from build123d import *


with BuildPart() as part:
    # 草图1 → 旋转1 (revolve)
    with BuildSketch(Plane.XY, mode=Mode.PRIVATE) as revolve_1_sk:
        Polygon((0, 0), (0, 42), (11.5, 42), (12.5, 40.267949192), (12.5, 0.267949192), (12, 0.267949192), (12, -0.732050808), (7.5, -0.732050808), (7.5, -22.732050808), (6.5, -23.732050808), (0, -23.732050808), align=None)
    revolve(revolve_1_sk.sketch.rotate(Axis((0, 0, 0), (0, 1, 0)), 90), axis=Axis((0, 0, 0), (0, 1, 0)))


solid = part.part
The listing builds one solid part. Answer for the finished solid, in the listing's coordinates (mm). A direction names the side the tool comes from. Round coordinates to 2 decimals unless told otherwise and drop trailing zeros. Write each loop counter-clockwise with the first axis right and the second up, starting at its lowest first coordinate (ties: lowest second). Pieces come first, ordered by that corner, then holes. Notation, with made-up numbers: (31.25, 24.5) - (67.25, 24.5) arc R28 ccw to (67.25, 50.5) - close; hole circle Ø8 at (7, -10.75). An arc over 180 degrees is marked (long way). Use one line per item in the form item = value. Start each with the question number.
Item 1: A tool of negligible diameter and unlimited length cuts with its end or side. For faces 3 (the cylindrical face through (-6.324, -11.886, -4.032)), 4 (the cylindrical face through (-3.755, 19.988, -11.923)), from which of +Z, -Z, +X, -X, +Y, -Y can it reach the whole face along a straight path? Write none if from no direction.
Item 2: A cutting plane is placed at A-A (x = 0). Write down the section's boundary in (y, z).
Item 3: A cutting plane is placed at B-B (z = 0). Write down the section's boundary in (x, y), plus the area to 3 significant figures.
Item 4: Find the intervals of material crossed by line 1 (Y direction, x = -6.5, z = -7.5); line 2 (Z direction, x = -0.5, y = 19); line 3 (X direction, y = 23.5, z = 6.5), in increasing order. Write a range as [from, to].
Item 5: A cutting plane is placed at D-D (y = -11). Write down the section's boundary in (x, z), plus the area to 3 significant figures.
Item 6: A cutting plane is placed at C-C (y = 17). Write down the section's boundary in (x, z), plus the area to 3 significant figures.
Item 7: Determine the mould class of faces 1 (the cylindrical face through (-3.604, -0.239, -11.446)), 2 (the flat face through (0, -23.732, 0)) for opening direction Z: +Z half, -Z half, draft (parallel to the pull), parting line (faces both ways), or undercut.
Item 8: Flat-ended cylindrical pins translate along their axes: pin 1 Ø1.5 at (y, z) = (-6, -9) entering from -X; pin 2 Ø4 at (x, z) = (-7, -3) entering from -Y; pin 3 Ø6 at (x, z) = (1.5, 9.5) entering from -Y; pin 4 Ø1.5 at (y, z) = (23.5, 10) entering from -X. Find the tip coordinate at first contact, or state that the pin passes through.
The answers:
q1.face_3 = -Y
q1.face_4 = +Y, -Y
q2.outline = (-23.73, -6.5) - (-22.73, -7.5) - (-0.73, -7.5) - (-0.73, -12) - (0.27, -12) - (0.27, -12.5) - (40.27, -12.5) - (42, -11.5) - (42, 11.5) - (40.27, 12.5) - (0.27, 12.5) - (0.27, 12) - (-0.73, 12) - (-0.73, 7.5) - (-22.73, 7.5) - (-23.73, 6.5) - close
q3.outline = (-12.5, 0.27) - (-12, 0.27) - (-12, -0.73) - (-7.5, -0.73) - (-7.5, -22.73) - (-6.5, -23.73) - (6.5, -23.73) - (7.5, -22.73) - (7.5, -0.73) - (12, -0.73) - (12, 0.27) - (12.5, 0.27) - (12.5, 40.27) - (11.5, 42) - (-11.5, 42) - (-12.5, 40.27) - close
q3.area = 1,410 mm^2
q4.line_1 = [-0.73, 42]
q4.line_2 = [-12.49, 12.49]
q4.line_3 = [-10.68, 10.68]
q5.outline = circle Ø15 at (0, 0)
q5.area = 177 mm^2
q6.outline = circle Ø25 at (0, 0)
q6.area = 491 mm^2
q7.face_1 = parting line
q7.face_2 = draft
q8.pin_1 = through
q8.pin_2 = -23.73
q8.pin_3 = -23.61
q8.pin_4 = -8.41
